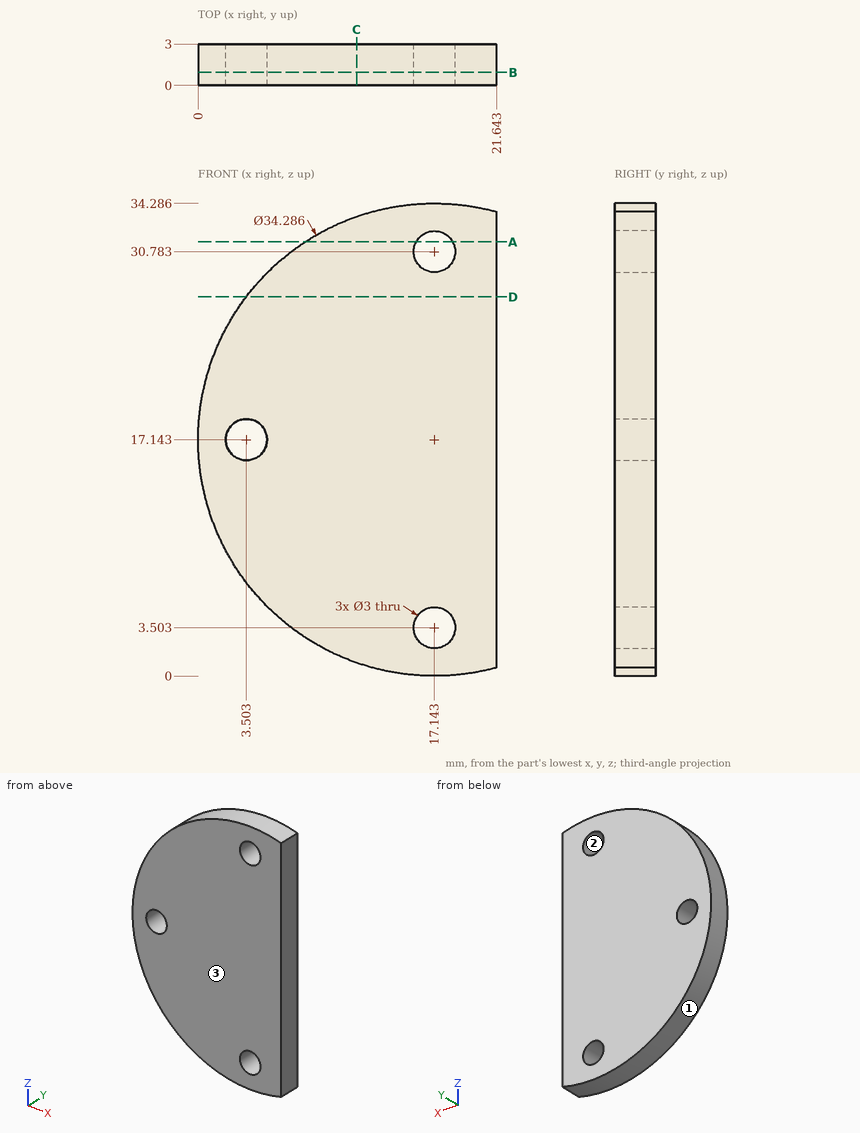
Here's the drawing with two shaded views (mm, measured from the low corner). I have some questions. Round coordinates to 2 decimals unless told otherwise and drop trailing zeros. Write each loop counter-clockwise with the first axis right and the second up, starting at its lowest first coordinate (ties: lowest second). Pieces come first, ordered by that corner, then holes. Notation, with made-up numbers: M 25,30.25 L 47,30.25 A19 ccw 47,57.25 Z; hole C 55,71 d4. An arc over 180 degrees is marked long. Answer in a Markdown table with one row per item. Add a question column.
Q1. Imagine slicing it at C-C (x = 11.5). Please give me the cut outline in (y, z) (1 decimal).
Q2. If I drill on line 1 (Z direction, x = 18, y = 0.15) (1 decimal); line 2 (Z direction, x = 16, y = 1.15) (1 decimal); line 3 (Z direction, x = 2.25, y = 0.6) (1 decimal), over which ranges is the centre line in solid material (lowest first)? Write a range as from..to.
Q3. Imagine slicing it at B-B (y = 0.95). Please give me the cut outline in (x, z) (1 decimal).
Q4. If we mould it in two halves opening along Z, with no side actions, what happens to the marked faces 1, 2 and 3? For each: +Z half, -Z half, draft (parallel to the pull), parting line (faces both ways), or undercut.
Q5. Imagine slicing it at A-A (z = 31.5). Please give me the cut outline in (x, y) (1 decimal).
Q6. Will this pin go through, and if not, where does the flat tip stop? pin 1 Ø2.5 at (x, z) = (17.14, 3.5) entering from +Y.
Q7. Imagine slicing it at D-D (z = 27.5). Please give me the cut outline in (x, y).
Values:
| question | item | result |
|---|---|---|
| 1 | outline | M 0,1 L 3,1 L 3,33.3 L 0,33.3 Z |
| 2 | line 1 | 0..2.3, 4.7..29.6, 32..34.3 |
| 2 | line 2 | 0..2.5, 4.5..29.8, 31.8..34.2 |
| 2 | line 3 | 8.7..16.3, 18..25.6 |
| 3 | outline | M 21.6,0.6 L 21.6,33.7 A17.1 ccw long Z; hole C 3.5,17.1 d3; hole C 17.1,3.5 d3; hole C 17.1,30.8 d3 |
| 4 | face 1 | parting line |
| 4 | face 2 | undercut |
| 4 | face 3 | draft |
| 5 | outline | M 7.8,0 L 15.8,0 L 15.8,3 L 7.8,3 Z; M 18.5,0 L 21.6,0 L 21.6,3 L 18.5,3 Z |
| 6 | pin 1 | through |
| 7 | outline | M 3.48,0 L 21.64,0 L 21.64,3 L 3.48,3 Z |
